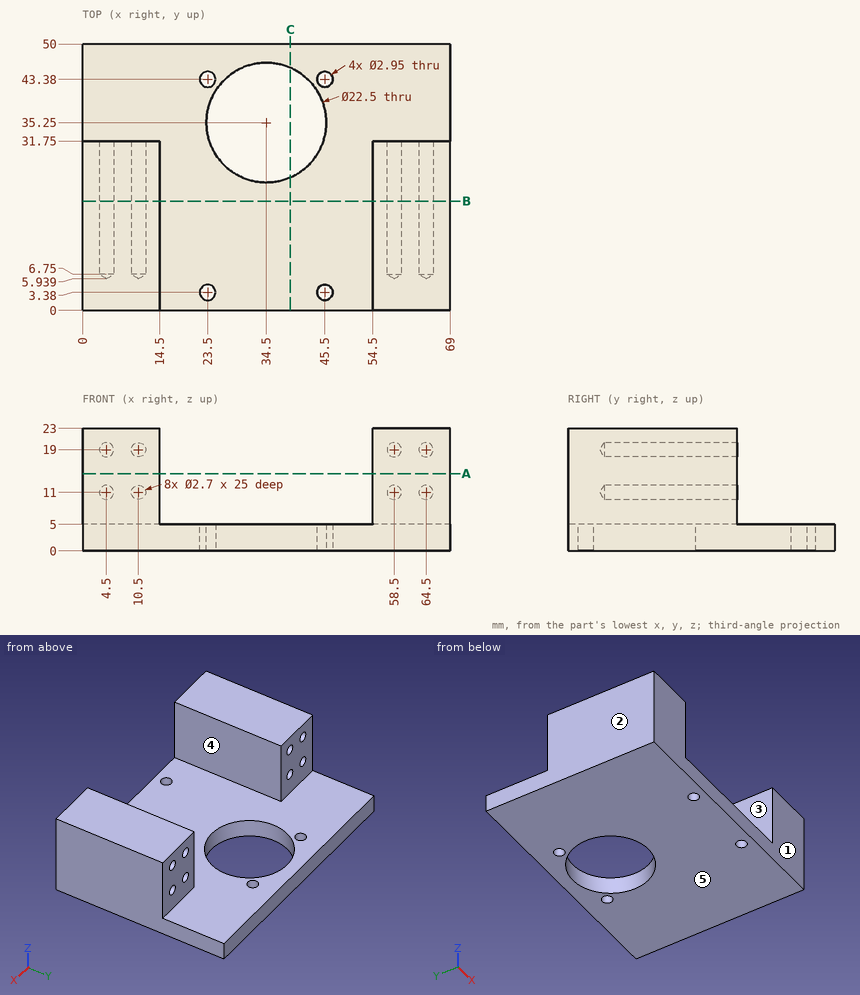
The figure shows three views and two pictorial views of one solid part (mm, origin at its lowest corner). Answer the questions. A direction names the side the tool comes from. Round coordinates to 2 decimals unless told otherwise and drop trailing zeros. Loops run counter-clockwise (first coordinate to the right, second up) from the corner with the lowest first, then second, coordinate; pieces in that order, holes last. Notation, with made-up numbers: (83.5, 66.5) - (120.5, 66.5) arc R21 cw to (120.5, 100.5) - close; hole circle Ø7 at (-39.75, 26). An arc over 180 degrees is marked (long way). One line per question, with ' | ' between items. Start each with the question number.
Q1. Section A-A on z = 14.5 is taken. Give the vertices of the cut face in (x, y).
Q2. For a pull along X with two mould halves and no side action, classify the marked faces 1, 2 and 3 as +X half, -X half, draft (parallel to the pull), parting line (faces both ways), or undercut.
Q3. Find the intervals of material crossed by L1, parallel to Z at x = 64.5, y = 21; L2, parallel to X at y = 24.25, z = 11; L3, parallel to Z at x = 59.5, y = 9 (1 decimal), in increasing order.
Q4. For the marked faces 4 and 5, determine the directions among +Z, -Z, +X, -X, +Y, -Y from which every point of the face is accessible in a straight line to the end or side of a thin tool.
Q5. Section C-C on x = 39 is taken. Give the vertices of the cut face in (y, z).
Q6. Section B-B on y = 20.5 is taken. Count the separate pieces of the cut face and the enclosed holes in it, plus the area to 3 significant figures.
Q7. Flat-ended cylindrical pins translate along their axes: pin 1 (8 mm diameter, centred on x = 61.5, y = 39.5, fed in from +Z); pin 2 (10 mm diameter, centred on x = 41.5, z = 7, fed in from -Y); pin 3 (4.5 mm diameter, centred on x = 64.5, z = 11, fed in from +Y). Find the tip coordinate at first contact, or state that the pin passes through.
Established:
1) outline: (0, 0) - (14.5, 0) - (14.5, 31.75) - (0, 31.75) - close; (54.5, 0) - (69, 0) - (69, 31.75) - (54.5, 31.75) - close
2) face 1: draft | face 2: -X half | face 3: undercut
3) L1: 0 to 9.65, 12.35 to 17.65, 20.35 to 23 | L2: 0 to 3.15, 5.85 to 9.15, 11.85 to 14.5, 54.5 to 57.15, 59.85 to 63.15, 65.85 to 69 | L3: 0 to 10.1, 11.9 to 18.1, 19.9 to 23
4) face 4: +Z, +Y, -Y | face 5: -Z, +X, -X, +Y, -Y
5) outline: (0, 0) - (24.94, 0) - (24.94, 5) - (0, 5) - close; (45.56, 0) - (50, 0) - (50, 5) - (45.56, 5) - close
6) separate pieces: 1 | enclosed holes: 8 | area: 821 mm²
7) pin 1: z = 5 | pin 2: y = 0 | pin 3: y = 31.75
